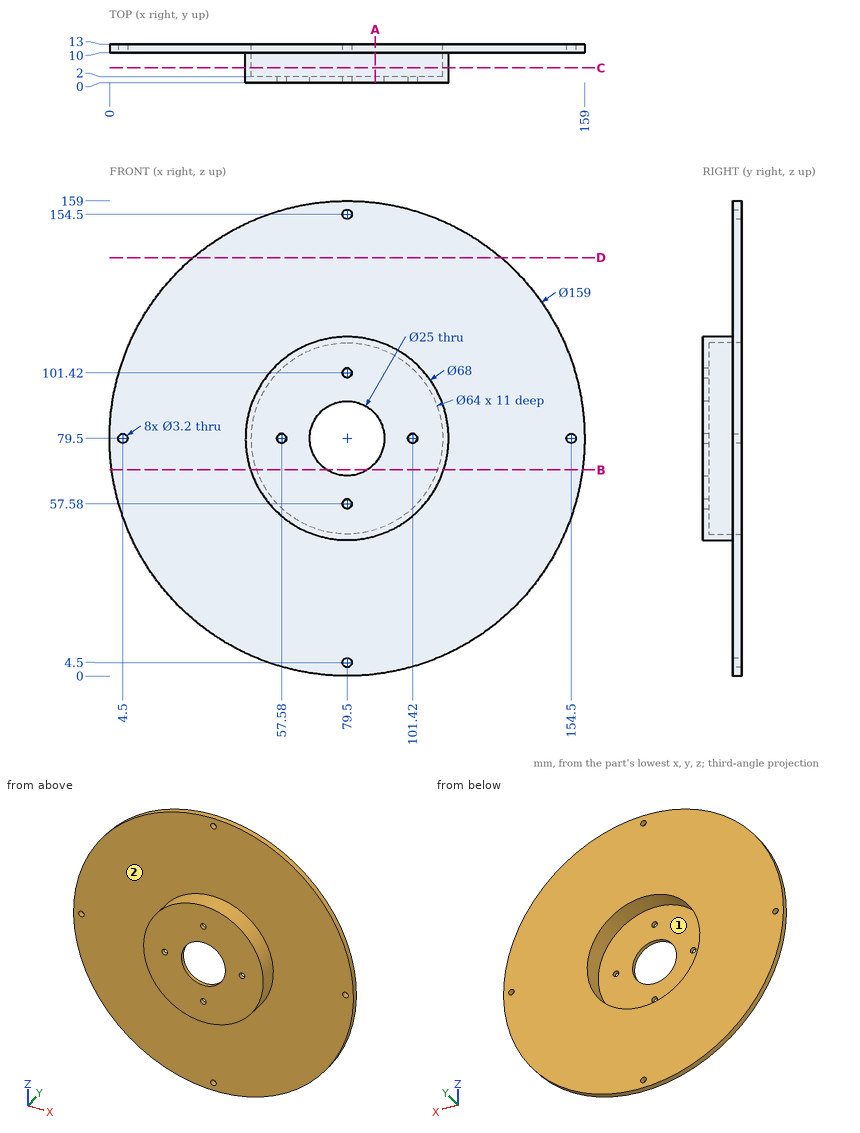
Study the drawing (mm; zero at the part's minimum x, y, z) and answer. Coordinates: 2 decimals unless noted, no trailing zeros. Loops run counter-clockwise (first coordinate to the right, second up) from the corner with the lowest first, then second, coordinate; pieces in that order, holes last. Notation, with made-up numbers: (36, 83) -> (94, 83) arc R28 ccw to (94, 110) -> close; hole circle Ø11 at (67.5, 69). An arc over 180 degrees is marked (long way). Write item = value, one per line. Start each with the question number.
1) The part is cut by section C-C, the plane y = 5. Determine the outline of the cut face in (x, z).
2) The mould has two halves that part along Y. Classify the marked faces 1 and 2: pulls with the +Y half, pulls with the -Y half, needs draft (parallel to the pull), parting line crosses it, or undercut.
3) Find the intervals of material crossed by L1, parallel to X at y = 10.75, z = 79.5; L2, parallel to X at y = 0.8, z = 79.5; L3, parallel to Y at x = 105, z = 79, in increasing order. Write a range as from..to.
4) Given P1, Ø2.5, axis at x = 79.5, z = 4.5, coming from the +Y side; P2, Ø4, axis at x = 57.58, z = 79.5, coming from the +Y side; P3, Ø8, axis at x = 67, z = 88, coming from the -Y side; P4, Ø1, axis at x = 61, y = 4, coming from the -Z side, each flat-ended and moving along its own axis, determine where each tip first touches the part or whether it passes through.
5) The part is cut by section D-D, the plane z = 140. Determine the outline of the cut face in (x, y).
6) The part is cut by section A-A, the plane x = 89. Determine the outline of the cut face in (y, z), plus the area to 3 significant figures.
7) The part is cut by section B-B, the plane z = 69. Determine the outline of the cut face in (x, y), plus the area to 3 significant figures.
Result:
q1.outline = circle Ø68 at (79.5, 79.5); hole circle Ø64 at (79.5, 79.5)
q2.face_1 = pulls with the +Y half
q2.face_2 = pulls with the -Y half
q3.L1 = 0..2.9, 6.1..47.5, 111.5..152.9, 156.1..159
q3.L2 = 45.5..55.98, 59.18..67, 92..99.82, 103.02..113.5
q3.L3 = 0..2
q4.P1 = through
q4.P2 = 2
q4.P3 = 0
q4.P4 = 50.66
q5.outline = (27.92, 10) -> (131.08, 10) -> (131.08, 13) -> (27.92, 13) -> close
q6.outline = (0, 46.85) -> (10, 46.85) -> (10, 0.57) -> (13, 0.57) -> (13, 48.94) -> (2, 48.94) -> (2, 71.38) -> (0, 71.38) -> close; (0, 87.62) -> (2, 87.62) -> (2, 110.06) -> (13, 110.06) -> (13, 158.43) -> (10, 158.43) -> (10, 112.15) -> (0, 112.15) -> close
q6.area = 422 mm²
q7.outline = (0.7, 10) -> (47.16, 10) -> (47.16, 0) -> (72.72, 0) -> (72.72, 2) -> (49.27, 2) -> (49.27, 13) -> (0.7, 13) -> close; (86.28, 0) -> (111.84, 0) -> (111.84, 10) -> (158.3, 10) -> (158.3, 13) -> (109.73, 13) -> (109.73, 2) -> (86.28, 2) -> close
q7.area = 427 mm²
